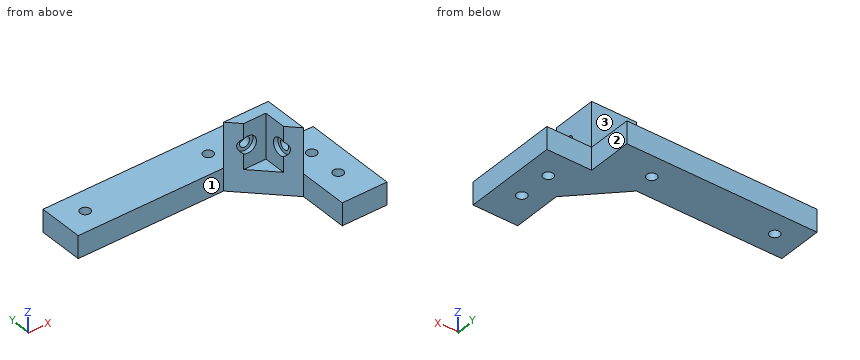
from build123d import *

# Parameters (mm, degrees)
F0_R      = 2.25
F1_DEPTH  = 10
F3_DEPTH  = 20
F4_R      = 2.25
F5_DEPTH  = 5
F6_R      = 2.25
F7_DEPTH  = 10
F8_R      = 3.75
F9_DEPTH  = 2
F10_R     = 3.75
F11_DEPTH = 2


with BuildPart() as f1:
    # F0 (on Top) → F1 (new body)
    with BuildSketch(Plane.XY):
        Polygon((-20, 20), (0, 0), (0, -22), (20, -22), (20, 20), (0, 20), (0, 40), (-85, 40), (-85, 20), align=None)
        with Locations((10, -7)):
            Circle(F0_R, mode=Mode.SUBTRACT)
        with Locations((10, 8)):
            Circle(F0_R, mode=Mode.SUBTRACT)
        with Locations((-74, 30)):
            Circle(F0_R, mode=Mode.SUBTRACT)
        with Locations((-19, 30)):
            Circle(F0_R, mode=Mode.SUBTRACT)
    extrude(amount=F1_DEPTH)

    # F2 (on face) → F3 (join)
    with BuildSketch(Plane.XY.offset(10)):
        Polygon((0, 0), (0, 20), (-20, 20), (-15, 15), (-10, 15), (-5, 15), (-5, 10), (-5, 5), align=None)
    extrude(amount=F3_DEPTH)

    # F4 (on face) → F5 (cut)
    with BuildSketch(Plane.YZ):
        with Locations((7, 20)):
            Circle(F4_R)
    extrude(amount=-F5_DEPTH, mode=Mode.SUBTRACT)

    # F6 (on face) → F7 (cut)
    with BuildSketch(Plane(origin=(0, 20, 0), x_dir=(-1, 0, 0), z_dir=(0, 1, 0))):
        with Locations((13, 20)):
            Circle(F6_R)
    extrude(amount=-F7_DEPTH, mode=Mode.SUBTRACT)

    # F8 (on face) → F9 (cut)
    with BuildSketch(Plane.XZ.offset(-15)):
        with Locations((-13, 20)):
            Circle(F8_R)
    extrude(amount=-F9_DEPTH, mode=Mode.SUBTRACT)

    # F10 (on face) → F11 (cut)
    with BuildSketch(Plane(origin=(-5, 0, 0), x_dir=(0, -1, 0), z_dir=(-1, 0, 0))):
        with Locations((-7, 20)):
            Circle(F10_R)
    extrude(amount=-F11_DEPTH, mode=Mode.SUBTRACT)


solid = f1.part
For this review, take the finished solid that the model builds, in its own axes (mm). Face numbers are marked on the shaded views. A direction names the side the tool comes from. Round coordinates to 2 decimals unless told otherwise and drop trailing zeros. Loops run counter-clockwise (first coordinate to the right, second up) from the corner with the lowest first, then second, coordinate; pieces in that order, holes last. Notation, with made-up numbers: (7.5, 14.25) - (16.5, 14.25) arc R20 ccw to (16.5, 37.25) - close; hole circle Ø11 at (82, 73). An arc over 180 degrees is marked (long way). One line per item, written item: value. Start each with the question number.
Item 1: Take a section at B-B (z = 20). Give the boundary of the cut face in (x, y), plus the area to 3 significant figures.
Item 2: For the marked faces 1, 2 and 3, list the 3-axis set-ups (+Z, -Z, +X, -X, +Y, -Y) from which the entire face can be reached by the end or side of a thin tool; tool diameter is ignored.
Item 3: Take a section at A-A (y = 30). Give the boundary of the cut face in (x, z), plus the area to 3 significant figures.
Item 4: Clearance check with flat-ended pins moving along their axes: pin 1 Ø8 at (x, z) = (-10, 23.5) entering from -Y; pin 2 Ø12 at (y, z) = (7, 20) entering from -X; pin 3 Ø4 at (y, z) = (7, 19) entering from -X; pin 4 Ø2.5 at (x, y) = (-74, 30) entering from -Z. State where each tip first meets the part, or that it passes through.
Item 5: For L1, parallel to Y at x = -74, z = 2.75; L2, parallel to Y at x = 10, z = 5.75; L3, parallel to Z at x = -13, y = 19.35, list the stretches that pass through material, from the lowest coordinate up.
Item 6: Take a section at C-C (y = -7). Give the boundary of the cut face in (x, z).
Item 7: Take a section at D-D (x = -13). Give the boundary of the cut face in (y, z).
Answer below:
1. outline: (-20, 20) - (-16.75, 16.75) - (-16.75, 17) - (-15.25, 17) - (-15.25, 20) - close; (-10.75, 17) - (-9.25, 17) - (-9.25, 15) - (-5, 15) - (-5, 10.75) - (-3, 10.75) - (-3, 9.25) - (0, 9.25) - (0, 20) - (-10.75, 20) - close; (-3.25, 3.25) - (0, 0) - (0, 4.75) - (-3, 4.75) - (-3, 3.25) - close
1. area: 96.1 mm2
2. face 1: +Z, -Z, -X, -Y
2. face 2: +Z, -Z, +X, +Y
2. face 3: +Z, +X, -X, +Y
3. outline: (-85, 0) - (-76.25, 0) - (-76.25, 10) - (-85, 10) - close; (-71.75, 0) - (-21.25, 0) - (-21.25, 10) - (-71.75, 10) - close; (-16.75, 0) - (0, 0) - (0, 10) - (-16.75, 10) - close
3. area: 760 mm2
4. pin 1: stops at y = 15
4. pin 2: stops at x = -5
4. pin 3: stops at x = -3
4. pin 4: passes through
5. L1: y = 20 to 27.75, 32.25 to 40
5. L2: y = -22 to -9.25, -4.75 to 5.75, 10.25 to 20
5. L3: z = 0 to 17.75, 22.25 to 30
6. outline: (0, 0) - (7.75, 0) - (7.75, 10) - (0, 10) - close; (12.25, 0) - (20, 0) - (20, 10) - (12.25, 10) - close
7. outline: (13, 0) - (40, 0) - (40, 10) - (20, 10) - (20, 17.75) - (17, 17.75) - (17, 16.25) - (15, 16.25) - (15, 10) - (13, 10) - close; (15, 23.75) - (17, 23.75) - (17, 22.25) - (20, 22.25) - (20, 30) - (15, 30) - close
